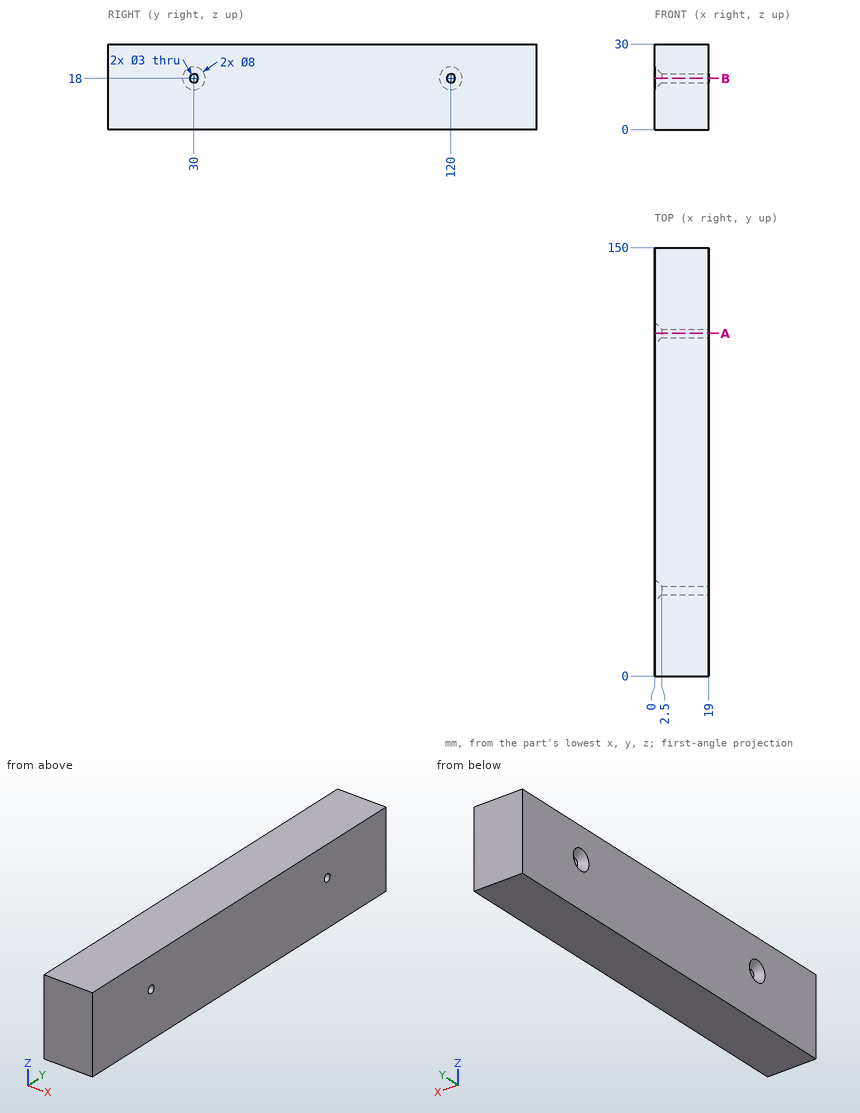
Source: three-view drawing plus pictorial views. Frame: mm from the lowest corner of the part. Give positions to 0.01 mm unless a question says otherwise; leave off trailing zeros. Order: outer loops, then holes, each group sorted by start corner. A loop starts at its lowest first (then second) coordinate and runs counter-clockwise, first axis right, second up. Notation, with made-up numbers: (22, 3) - (28, 3) arc R17 cw to (28, 33) - close; hole circle Ø1 at (-21.5, -4). An arc over 180 degrees is marked (long way). Answer as a JSON object with one key per item and string values. Group by question number.
Q1. Cut plane A-A, the plane y = 120. Output: boundary loops of the cut face in (x, z), then the cut area to 3 significant figures.
Q2. First-contact query: pin 1 Ø2.5 at (y, z) = (30, 18) entering from +X; pin 2 Ø3.5 at (y, z) = (120, 18) entering from -X. Flat tips, straight axial feed; report the tip coordinate or a pass-through.
Q3. Line query: probe 1 along Y at (x, z) = (9, 18.25); probe 2 along Z at (x, y) = (15.25, 30); probe 3 along Y at (x, z) = (13.75, 19.25). Output: solid intervals per line, ascending.
Q4. Cut plane B-B, the plane z = 18. Output: boundary loops of the cut face in (x, y).
Results:
{
 "1": {"outline": "(0, 0) - (19, 0) - (19, 16.5) - (2.5, 16.5) - (0, 14) - close; (0, 22) - (2.5, 19.5) - (19, 19.5) - (19, 30) - (0, 30) - close", "area": "507 mm^2"},
 "2": {"pin 1": "through", "pin 2": "x = 2.25"},
 "3": {"probe 1": "0 to 28.52, 31.48 to 118.52, 121.48 to 150", "probe 2": "0 to 16.5, 19.5 to 30", "probe 3": "0 to 29.17, 30.83 to 119.17, 120.83 to 150"},
 "4": {"outline": "(0, 0) - (19, 0) - (19, 28.5) - (2.5, 28.5) - (0, 26) - close; (0, 34) - (2.5, 31.5) - (19, 31.5) - (19, 118.5) - (2.5, 118.5) - (0, 116) - close; (0, 124) - (2.5, 121.5) - (19, 121.5) - (19, 150) - (0, 150) - close"}
}
